Read the model definition and answer for the solid it produces. Units are mm, in the model's axes. A direction names the side the tool comes from. Give positions to 0.01 mm unless a question says otherwise; leave off trailing zeros. Return JSON: item names as keys, results as strings. Group by question number.
Autodesk Inventor part; units mm, degrees
ref_plane "height_panel" through (0, 110, 0) normal (0, 1, 0) x (1, 0, 0)
ref_plane "Work Plane2" through (0, 0, -15.8234) normal (-1, 0, 0) x (0, 0, 1)
ref_plane "YZ Plane" through (0, 0, 0) normal (1, 0, 0) x (0, 1, 0)
sketch "Sketch1" plane through (0, 0, 0) normal (0, 1, 0) x (-1, 0, 0)
  line L0 (18, 18) -> (-18, 18)
  line L1 (-18, 18) -> (-18, -18)
  line L2 (-1.0844, -18) -> (0, -18)
  line L3 (18, -18) -> (18, 18)
  line L4 (0, 31.7221) -> (0, -30.6703)
  line L5 (20.2298, 0) -> (-39.3416, 0)
  line L6 (18, 62) -> (-19.0844, 62) construction
  arc A0 (0, -18) -> (18, -15.8234) centre (-0.5422, 62) ccw
  arc A1 (-18, -16.0738) -> (-1.0844, -18) centre (-0.5422, 62) ccw
  circle A2 centre (0, 0) radius 5.1
  dimension "d0" = 36
  dimension "d1" = 36
  dimension "d2" = 80
  dimension "d6" = 10.2
extrude "Extrusion1" add sketch "Sketch1" along normal blind 10
extrude "Extrusion2" cut sketch "Sketch1" along normal through all contours A2 L5 L4 | L4 L5 A2 | A2 L4 L5 | L4 A2 L5
sketch "Sketch2" plane through (0, 10, 0) normal (0, 1, 0) x (1, 0, 0)
  circle A0 centre (0, 0) radius 5.1 construction
  line L0 (-18, -18) -> (18, -18) construction
  line L1 (18, -18) -> (18, 16.0738) construction
  arc A1 (18, 16.0738) -> (1.0844, 18) centre (0.5422, -62) ccw construction
  line L2 (1.0844, 18) -> (0, 18) construction
  arc A2 (0, 18) -> (-18, 15.8234) centre (0.5422, -62) ccw construction
  line L3 (-18, 15.8234) -> (-18, -18) construction
  line L4 (18, -18) -> (10, -18)
  line L5 (10, -18) -> (10, 15.8234)
  line L6 (10, 15.8234) -> (18, 15.8234)
  line L7 (18, 15.8234) -> (18, -18)
  dimension "d9" = 8
ref_plane "height_panel" through (0, 110, 0) normal (0, 1, 0) x (1, 0, 0)
sketch "Sketch3" plane through (0, 110, 0) normal (0, 1, 0) x (1, 0, 0)
  line L0 (15, 60) -> (30, 60)
  line L1 (30, 60) -> (30, 170)
  line L2 (30, 170) -> (15, 170)
  line L3 (15, 170) -> (15, 60)
  line L4 (0, -34.344) -> (0, 41.1374) construction
  circle A0 centre (0, 0) radius 5.1 construction
  line L5 (0, 0) -> (37.0806, 0) construction
  line L6 (0, 0) -> (-113.2425, 196.1417) construction
  line L7 (0, 0) -> (113.2425, 196.1417) construction
  dimension "d15" = 15
  dimension "d16" = 110
  dimension "d17" = 30
  dimension "d18" = 0
  dimension "d20" = 60
  dimension "d23" = 60
loft "support_panel" add profiles "Sketch2", "Sketch3"
ref_plane "Work Plane2" through (0, 0, -15.8234) normal (-1, 0, 0) x (0, 0, 1)
mirror "Mirror1" about plane through (0, 0, -15.8234) normal (-1, 0, 0) of "support_panel"
sketch "Sketch4" plane through (0, 0, -15.8234) normal (-1, 0, 0) x (0, 0, 1)
  line L0 (0, 10) -> (33.8234, 10) construction
  line L1 (33.8234, 10) -> (-44.1766, 110) construction
  line L2 (-154.1766, 110) -> (-44.1766, 110) construction
  line L3 (0, 10) -> (-154.1766, 110) construction
  line L4 (0, 10) -> (-154.1766, 110)
  line L5 (-61.6706, 50) -> (-42.7634, 108.1882)
  line L6 (33.8234, 10) -> (-44.1766, 110)
  line L7 (-3.2973, 57.5907) -> (-15.4177, 20)
  line L8 (-42.7634, 108.1882) -> (-3.2973, 57.5907)
  line L9 (-61.6706, 50) -> (-15.4177, 20)
  point P0 (15.8234, 0)
  dimension "d24" = 60
  dimension "d25" = 90
extrude "Extrusion3" add sketch "Sketch4" along normal mid plane 38
sketch "Sketch5" plane through (0, 0, -15.8234) normal (-1, 0, 0) x (0, 0, 1)
  line L0 (-20.1302, 94) -> (-176.0391, 94) construction
  line L1 (-154.1766, 110) -> (-44.1766, 110) construction
  line L2 (-18.8309, 102) -> (-169.7053, 102) construction
  line L3 (33.8234, 10) -> (-44.1766, 110) construction
  line L4 (-44.1766, 110) -> (-44.1766, 74.3483) construction
  line L5 (-71.6766, 137.3856) -> (-71.6766, 103.9302) construction
  line L6 (-126.6766, 137.3856) -> (-126.6766, 97.2716) construction
  line L7 (-44.1766, 110) -> (-154.1766, 110) construction
  line L8 (-99.1766, 110) -> (-99.1766, 73.2356) construction
  circle A0 centre (-71.6766, 102) radius 2.5 construction
  line L9 (-69.1766, 104.5) -> (-74.1766, 104.5)
  line L10 (-74.1766, 104.5) -> (-74.1766, 99.5)
  line L11 (-74.1766, 99.5) -> (-69.1766, 99.5)
  line L12 (-69.1766, 99.5) -> (-69.1766, 104.5)
  circle A1 centre (-126.6766, 102) radius 2.5 construction
  line L13 (-129.1766, 104.5) -> (-124.1766, 104.5)
  line L14 (-124.1766, 104.5) -> (-124.1766, 99.5)
  line L15 (-124.1766, 99.5) -> (-129.1766, 99.5)
  line L16 (-129.1766, 99.5) -> (-129.1766, 104.5)
  line L17 (-44.1766, 110) -> (-31.6966, 94)
  line L18 (0, 10) -> (-154.1766, 110)
  line L19 (-129.5083, 94) -> (-154.1766, 110)
  line L20 (-154.1766, 110) -> (-44.1766, 110)
  line L21 (-31.6966, 94) -> (-129.5083, 94)
  line L22 (-44.1766, 94) -> (-129.5083, 94)
  line L23 (-44.1766, 94) -> (-44.1766, 84)
  line L24 (-44.1766, 84) -> (-114.0907, 84)
  line L25 (-114.0907, 84) -> (-129.5083, 94)
  line L26 (-44.1766, 94) -> (-129.5083, 94)
  point P0 (15.8234, 0)
  dimension "d28" = 16
  dimension "d29" = 8
  dimension "d30" = 55
  dimension "d31" = 5
  dimension "d40" = 10
extrude "Extrusion5" add sketch "Sketch5" along normal mid plane 60 contours L17 L21 L18 L20
extrude "installation_rack" cut sketch "Sketch5" along normal mid plane 25 contours L17 L21 L18 L20
extrude "Extrusion7" cut sketch "Sketch5" along normal through all both and the other way through all contours L12 L11 L10 L9 | L13 L14 L15 L16
extrude "Extrusion8" add sketch "Sketch5" along normal mid plane 30 contours L23 L24 L18 L21
properties part number "PRING_vertical_bar"
1. Flat-ended cylindrical pins translate along their axes: pin 1 Ø5.5 at (x, z) = (21, -87.5) entering from -Y; pin 2 Ø5 at (x, z) = (-6.5, -50.5) entering from +Y; pin 3 Ø2.5 at (x, y) = (21.5, 101) entering from -Z. Find the tip coordinate at first contact, or state that the pin passes through.
2. Determine the mould class of faces 1 (the flat face through (21, 102, -140)), 2 (the flat face through (29.27, 100.11, -154.75)), 3 (the cylindrical face through (-2.4, 4.9, 4.5)) for opening direction Y: pulls with the +Y half, pulls with the -Y half, needs draft (parallel to the pull), parting line crosses it, or undercut.
3. Straight lines are drawn through the part: line 1 (X direction, y = 3.75, z = 0); line 2 (X direction, y = 8.5, z = -1.5). For each, find the intervals that lie inside material, in ascending order. Write a range as from..to.
4. Which of the six approach directions +Z, -Z, +X, -X, +Y, -Y give full straight-line access (tool end or side, diameter ignored) to faces 4 (the flat face through (21, 104.5, -87)), 5 (the flat face through (18, 5, 1)), 6 (the flat face through (29.48, 98.556, -51.074)), 7 (the cylindrical face through (-9.188, 4.93, -17.408))?
5. Section A-A on x = 25.5 is taken. State how many separate pieces and enclosed holes the cut face has, then the cut area to 3 significant figures.
Completed:
{
 "1": {"pin 1": "stops at y = 54.71", "pin 2": "stops at y = 94", "pin 3": "stops at z = -158.05"},
 "2": {"face 1": "undercut", "face 2": "pulls with the -Y half", "face 3": "needs draft"},
 "3": {"line 1": "x = -18..-5.1, 5.1..18", "line 2": "x = -18..-4.87, 4.87..18"},
 "4": {"face 4": "+X, -X", "face 5": "+Z, -Z, +X, -Y", "face 6": "+Z, +X, -X, +Y", "face 7": "-Z, -X, -Y"},
 "5": {"separate pieces": "1", "enclosed holes": "2", "area": "3,540 mm²"}
}
